Autodesk Inventor part; units mm, degrees
ref_plane "YZ Plane" through (0, 0, 0) normal (1, 0, 0) x (0, 1, 0)
ref_plane "XZ Plane" through (0, 0, 0) normal (0, 1, 0) x (-1, 0, 0)
ref_plane "XY Plane" through (0, 0, 0) normal (0, 0, 1) x (1, 0, 0)
sketch "Sketch1" plane through (0, 0, 0) normal (0, 0, 1) x (1, 0, 0)
  line L0 (0, 0) -> (68, 0)
  line L1 (68, 0) -> (68, -32)
  line L2 (68, -32) -> (0, -32)
  line L3 (0, -32) -> (0, 0)
  dimension "d0" = 68
  dimension "d1" = 32
extrude "Extrusion1" add sketch "Sketch1" along normal blind 23
shell "Shell1" thickness 2 removed faces 1 at (22.6667, -10.6667, 23)
sketch "Sketch5" plane through (2, -30, 2) normal (0, 0, 1) x (1, 0, 0)
  line L0 (-2, 30) -> (3, 30)
  line L1 (66, 30) -> (-2, 30)
  line L2 (3, 30) -> (3, 14)
  line L3 (3, 14) -> (3, 24.25)
  line L4 (3, 24.25) -> (60.5, 24.25)
  line L5 (60.5, 24.25) -> (60.5, 3.75)
  line L6 (60.5, 3.75) -> (3, 3.75)
  line L7 (3, 3.75) -> (3, 14)
  circle A0 centre (60.5, 24.25) radius 0.75
  circle A1 centre (60.5, 3.75) radius 0.75
  circle A2 centre (3, 24.25) radius 0.75
  circle A3 centre (3, 3.75) radius 0.75
  dimension "d5" = 5
  dimension "d6" = 16
  dimension "d7" = 10.25
  dimension "d8" = 57.5
  dimension "d9" = 20.5
  dimension "d10" = 1.5
  dimension "d11" = 1.5
  dimension "d12" = 1.5
  dimension "d13" = 1.5
extrude "Extrusion2" add sketch "Sketch5" along normal blind 3 contours A2 L4 L2 | L2 A2 | L4 A2 L2 | A0 L5 L4 | L4 L5 A0 | A3 L6 L7 | L7 L6 A3 | A1 L6 L5 | L5 L6 A1
sketch "Sketch6" plane through (0, -32, 0) normal (-1, 0, 0) x (0, 0, 1)
  line L0 (2, 30) -> (2, 2)
  line L1 (2, 16) -> (2, 21)
  line L2 (2, 21) -> (9, 21)
  line L3 (9, 21) -> (9, 11)
  line L4 (9, 11) -> (2, 11)
  line L5 (2, 11) -> (2, 16)
  point P0 (0, 32)
  point P1 (2, 11)
  dimension "d16" = 5
  dimension "d17" = 7
  dimension "d18" = 10
extrude "Extrusion3" cut sketch "Sketch6" against normal blind 10
properties part number "laatikko"
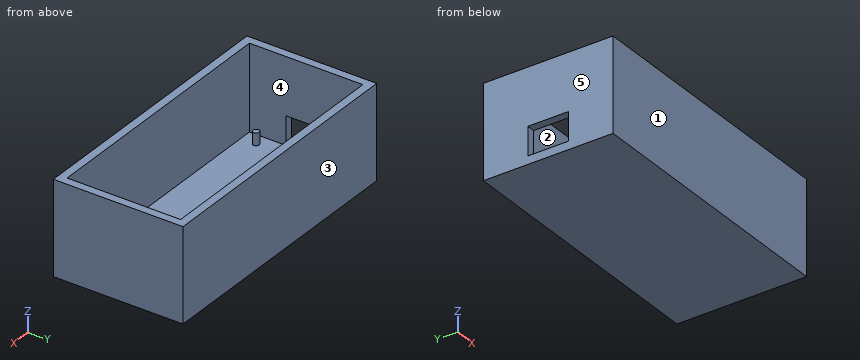
Verification items for the finished model (mm, model axes). Face numbers are marked on the shaded views. A direction names the side the tool comes from. Give positions to 0.01 mm unless a question says otherwise; leave off trailing zeros. Write each loop counter-clockwise with the first axis right and the second up, starting at its lowest first coordinate (ties: lowest second). Pieces come first, ordered by that corner, then holes.
(1) Cross-section at B-B (z = 10.75). Enter the section's corners in (x, y).
(2) Cross-section at D-D (y = -26.25). Enter the section's corners in (x, z), plus the area to 3 significant figures.
(3) Cross-section at C-C (x = 7.5). Enter the section's corners in (y, z).
(4) Mould release check, pull along Y, two halves, no side actions. Record for the marked faces 3, 4 and 5: +Y half, -Y half, draft (parallel to the pull), parting line (faces both ways), or undercut.
(5) Material ranges on line 1 (Y direction, x = 26.5, z = 11); line 2 (X direction, y = -7, z = 19.5); line 3 (Z direction, x = 43.5, y = -19.5), recorded low to high.
(6) Gauge pin test, flat ends, axial feed: pin 1 (5 mm diameter, centred on y = -16, z = 7, fed in from -X); pin 2 (1.6 mm diameter, centred on x = 62.5, y = -26.5, fed in from +Z); pin 3 (8 mm diameter, centred on x = 27.5, y = -16, fed in from +Z). Record the tip position at first contact, or that the pin passes through.
(7) Access from +Z, -Z, +X, -X, +Y, -Y to the whole of each face (thin tool, end or side, straight path). Record for the marked faces 1 and 2.
(8) Cross-section at A-A (y = -17). Enter the section's corners in (x, z).
Worked out:
1. outline: (0, -32) - (68, -32) - (68, 0) - (0, 0) - close; hole (2, -30) - (66, -30) - (66, -2) - (2, -2) - close
2. outline: (0, 0) - (68, 0) - (68, 23) - (66, 23) - (66, 2) - (63.25, 2) - (63.25, 5) - (61.75, 5) - (61.75, 2) - (5.75, 2) - (5.75, 5) - (4.25, 5) - (4.25, 2) - (2, 2) - (2, 23) - (0, 23) - close
2. area: 229 mm2
3. outline: (-32, 0) - (0, 0) - (0, 23) - (-2, 23) - (-2, 2) - (-30, 2) - (-30, 23) - (-32, 23) - close
4. face 3: +Y half
4. face 4: undercut
4. face 5: draft
5. line 1: y = -32 to -30, -2 to 0
5. line 2: x = 0 to 2, 66 to 68
5. line 3: z = 0 to 2
6. pin 1: stops at x = 0
6. pin 2: stops at z = 5
6. pin 3: stops at z = 2
7. face 1: +Z, -Z, +X, -X, -Y
7. face 2: +Z
8. outline: (0, 0) - (68, 0) - (68, 23) - (66, 23) - (66, 2) - (0, 2) - close; (0, 9) - (2, 9) - (2, 23) - (0, 23) - close
